from build123d import *

# Parameters (mm, degrees)
SKETCH1_W           = 317.5
SKETCH1_H           = 177.8
SKETCH1_R           = 3.175
SKETCH1_R_2         = 6.4135
SKETCH1_R_3         = 1.905
BOSS_EXTRUDE1_DEPTH = 3.175
SKETCH3_R           = 3.175
CUT_EXTRUDE2_DEPTH  = 182.974869488
SKETCH4_W           = 25.4
SKETCH4_H           = 177.8
CUT_EXTRUDE3_DEPTH  = 182.974869488
SKETCH5_R           = 5.08
CUT_EXTRUDE4_DEPTH  = 182.974869488
SKETCH6_R           = 1.8034
CUT_EXTRUDE5_DEPTH  = 182.974869488
SKETCH7_R           = 1.8415
CUT_EXTRUDE6_DEPTH  = 182.974869488


with BuildPart() as part:
    # Sketch1 → Boss-Extrude1 (new body)
    with BuildSketch(Plane(origin=(0, 0, 0), x_dir=(1, 0, 0), z_dir=(0, 1, 0))):
        Rectangle(SKETCH1_W, SKETCH1_H)
        with Locations(Location((-111.76, -12.7, 0), (0, 0, 270))):
            Circle(SKETCH1_R, mode=Mode.SUBTRACT)
        with Locations(Location((107.95, -6.35, 0), (0, 0, 270))):
            Circle(SKETCH1_R_2, mode=Mode.SUBTRACT)
        with Locations(Location((-129.032, 55.88, 0), (0, 0, 270))):
            Circle(SKETCH1_R_3, mode=Mode.SUBTRACT)
        with Locations(Location((-60.452, 55.88, 0), (0, 0, 270))):
            Circle(SKETCH1_R_3, mode=Mode.SUBTRACT)
        with Locations(Location((-129.032, 38.1, 0), (0, 0, 270))):
            Circle(SKETCH1_R_3, mode=Mode.SUBTRACT)
        with Locations(Location((-60.452, 38.1, 0), (0, 0, 270))):
            Circle(SKETCH1_R_3, mode=Mode.SUBTRACT)
    extrude(amount=BOSS_EXTRUDE1_DEPTH)

    # Sketch3 → Cut-Extrude2 (cut, through all)
    with BuildSketch(Plane(origin=(0, 0, 0), x_dir=(-1, 0, 0), z_dir=(0, -1, 0))):
        with Locations(Location((23.829539609, -72.39, 0), (0, 0, 90))):
            Circle(SKETCH3_R)
        with Locations(Location((-26.764302072, -67.818, 0), (0, 0, 90))):
            Circle(SKETCH3_R)
    extrude(amount=-CUT_EXTRUDE2_DEPTH, mode=Mode.SUBTRACT)

    # Sketch4 → Cut-Extrude3 (cut, through all)
    with BuildSketch(Plane(origin=(0, 3.175, 0), x_dir=(1, 0, 0), z_dir=(0, 1, 0))):
        with Locations((146.05, 0)):
            Rectangle(SKETCH4_W, SKETCH4_H)
    extrude(amount=-CUT_EXTRUDE3_DEPTH, mode=Mode.SUBTRACT)

    # Sketch5 → Cut-Extrude4 (cut, through all)
    with BuildSketch(Plane(origin=(0, 3.175, 0), x_dir=(1, 0, 0), z_dir=(0, 1, 0))):
        with Locations(Location((115.57, -38.1, 0), (0, 0, 270))):
            Circle(SKETCH5_R)
    extrude(amount=-CUT_EXTRUDE4_DEPTH, mode=Mode.SUBTRACT)

    # Sketch6 → Cut-Extrude5 (cut, through all)
    with BuildSketch(Plane.XZ):
        with Locations(Location((127, 69.85, 0), (0, 0, 270))):
            Circle(SKETCH6_R)
        with Locations(Location((127, 53.975, 0), (0, 0, 270))):
            Circle(SKETCH6_R)
        with Locations(Location((127, -53.975, 0), (0, 0, 270))):
            Circle(SKETCH6_R)
        with Locations(Location((127, -69.85, 0), (0, 0, 270))):
            Circle(SKETCH6_R)
    extrude(amount=-CUT_EXTRUDE5_DEPTH, mode=Mode.SUBTRACT)

    # Sketch7 → Cut-Extrude6 (cut, through all)
    with BuildSketch(Plane(origin=(0, 3.175, 0), x_dir=(1, 0, 0), z_dir=(0, 1, 0))):
        with Locations(Location((121.92, 39.6875, 0), (0, 0, 270))):
            Circle(SKETCH7_R)
        with Locations(Location((81.28, 39.6875, 0), (0, 0, 270))):
            Circle(SKETCH7_R)
        with Locations(Location((81.28, -26.9875, 0), (0, 0, 270))):
            Circle(SKETCH7_R)
        with Locations(Location((121.92, -26.9875, 0), (0, 0, 270))):
            Circle(SKETCH7_R)
        with Locations(Location((-88.265, -46.99, 0), (0, 0, 270))):
            Circle(SKETCH7_R)
        with Locations(Location((-67.31, -46.99, 0), (0, 0, 270))):
            Circle(SKETCH7_R)
        with Locations(Location((-87.3125, -37.1475, 0), (0, 0, 270))):
            Circle(SKETCH7_R)
        with Locations(Location((-68.2625, -37.1475, 0), (0, 0, 270))):
            Circle(SKETCH7_R)
        with Locations(Location((-87.3125, -8.5725, 0), (0, 0, 270))):
            Circle(SKETCH7_R)
        with Locations(Location((-88.265, 0, 0), (0, 0, 270))):
            Circle(SKETCH7_R)
        with Locations(Location((-67.31, 0, 0), (0, 0, 270))):
            Circle(SKETCH7_R)
    extrude(amount=-CUT_EXTRUDE6_DEPTH, mode=Mode.SUBTRACT)


solid = part.part
The model under review builds one solid part; all positions refer to its coordinate system, in mm. Coordinates: 2 decimals unless noted, no trailing zeros. Write each loop counter-clockwise with the first axis right and the second up, starting at its lowest first coordinate (ties: lowest second). Pieces come first, ordered by that corner, then holes. Notation, with made-up numbers: M -33,32 L 21,32 A18 cw 21,65 Z; hole C 22.25,62.25 d2. An arc over 180 degrees is marked long. Put each result on its own line as item: value.
1) Wall thickness on probe 1 along X at (y, z) = (1.5, 46.99); probe 2 along Z at (x, y) = (-130, 2.4); probe 3 along X at (y, z) = (1.2, 14): over which ranges is each line inside the solid? List them lowest first. Write a range as [from, to].
Computed:
probe 1: x = [-158.75, -90.11], [-86.42, -69.15], [-65.47, 133.35]
probe 2: z = [-88.9, -57.52], [-54.24, -39.74], [-36.46, 88.9]
probe 3: x = [-158.75, -114.66], [-108.86, 133.35]
2) Clearance check with flat-ended pins moving along their axes: pin 1 Ø7.5 at (x, z) = (-23.83, 72.39) entering from +Y (3 decimals); pin 2 Ø3.5 at (x, z) = (-129.032, -55.88) entering from +Y. State where each tip first meets the part, or that it passes through.
Computed:
pin 1: stops at y = 3.175
pin 2: passes through
3) Draft analysis for pull direction X (two halves, no side actions). For faces 1 (the flat face through (-15, 0, -1)), 2 (the cylindrical face through (119.003, 1.61, 34.356)), state which applies: released by +X, released by -X, zero draft, split by the parting line, or undercut.
Computed:
face 1: zero draft
face 2: undercut
4) Add section A-A on x = -111.76. Give the boundary of the cut face in (y, z) (3 decimals), then the cut area to 3 significant figures.
Computed:
outline: M 0,-88.9 L 3.175,-88.9 L 3.175,9.525 L 0,9.525 Z; M 0,15.875 L 3.175,15.875 L 3.175,88.9 L 0,88.9 Z
area: 544 mm2
